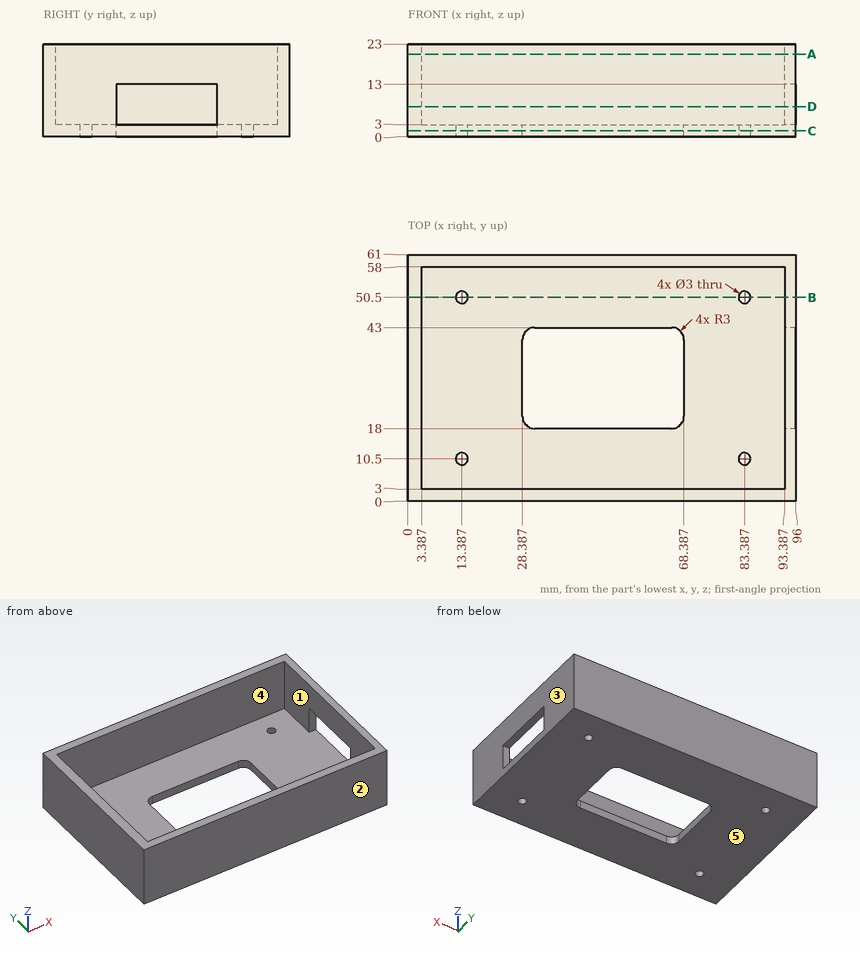
The figure shows three views and two pictorial views of one solid part (mm, origin at its lowest corner). Answer the questions. A direction names the side the tool comes from. Give positions to 0.01 mm unless a question says otherwise; leave off trailing zeros. Write each loop counter-clockwise with the first axis right and the second up, starting at its lowest first coordinate (ties: lowest second). Pieces come first, ordered by that corner, then holes. Notation, with made-up numbers: M -33,63.5 L 9,63.5 A27 cw 9,89.5 Z; hole C 46.25,66.25 d2. An arc over 180 degrees is marked long. Write each question's results on one line, items separated by ' | '.
Q1. Section D-D, the plane z = 7.5 is taken. Write down the section's boundary in (x, y).
Output values:
outline: M 0,0 L 96,0 L 96,18 L 93.39,18 L 93.39,3 L 3.39,3 L 3.39,58 L 93.39,58 L 93.39,43 L 96,43 L 96,61 L 0,61 Z
Q2. Section A-A, the plane z = 20.5 is taken. Write down the section's boundary in (x, y).
Output values:
outline: M 0,0 L 96,0 L 96,61 L 0,61 Z; hole M 3.39,3 L 93.39,3 L 93.39,58 L 3.39,58 Z
Q3. Section C-C, the plane z = 1.5 is taken. Write down the section's boundary in (x, y), then the cut area to 3 significant figures.
Output values:
outline: M 0,0 L 96,0 L 96,61 L 0,61 Z; hole C 13.39,10.5 d3; hole C 13.39,50.5 d3; hole M 28.39,21 A3 ccw 31.39,18 L 65.39,18 A3 ccw 68.39,21 L 68.39,40 A3 ccw 65.39,43 L 31.39,43 A3 ccw 28.39,40 Z; hole C 83.39,10.5 d3; hole C 83.39,50.5 d3 | area: 4,840 mm2
Q4. A tool of negligible diameter and unlimited length cuts with its end or side. For the marked faces 4 and 5, from which of +Z, -Z, +X, -X, +Y, -Y can it reach the whole face along a straight path? Write none if from no direction.
Output values:
face 4: +Z | face 5: -Z, +X, -X, +Y, -Y
Q5. Consider L1, parallel to X at y = 42, z = 16; L2, parallel to Y at x = 13.5, z = 5.5; L3, parallel to Y at x = 47.5, z = 1. Determine where each line is inside the solid, lowest interval first. Write a range as from..to.
Output values:
L1: 0..3.39, 93.39..96 | L2: 0..3, 58..61 | L3: 0..18, 43..61
Q6. Flat-ended cylindrical pins translate along their axes: P1, Ø1.8, axis at x = 83.39, y = 50.5, coming from the +Z side; P2, Ø5, axis at x = 13.39, y = 10.5, coming from the -Z side. Find the tip coordinate at first contact, or state that the pin passes through.
Output values:
P1: through | P2: z = 0
Q7. Section B-B, the plane y = 50.5 is taken. Write down the section's boundary in (x, z), then the cut area to 3 significant figures.
Output values:
outline: M 0,0 L 11.89,0 L 11.89,3 L 3.39,3 L 3.39,23 L 0,23 Z; M 14.89,0 L 81.89,0 L 81.89,3 L 14.89,3 Z; M 84.89,0 L 96,0 L 96,23 L 93.39,23 L 93.39,3 L 84.89,3 Z | area: 390 mm2
Q8. For a pull along X with two mould halves and no side action, classify the marked faces 1, 2 and 3 as released by +X, released by -X, zero draft, split by the parting line, or undercut.
Output values:
face 1: undercut | face 2: zero draft | face 3: released by +X
